Verification items for the finished model (mm, model axes). Coordinates: 2 decimals unless noted, no trailing zeros. Loops run counter-clockwise (first coordinate to the right, second up) from the corner with the lowest first, then second, coordinate; pieces in that order, holes last.
Q1. Sectioned sample at A-A (z = -85). Enter the section's corners in (x, y), then the cut area to 3 significant figures.
Q2. Go/stop test with flat-tipped pins: P1, Ø3, axis at y = 3.5, z = -5, coming from the +X side; P2, Ø3, axis at y = 2, z = -146.5, coming from the +X side; P3, Ø11.5, axis at x = -18, z = -125, coming from the -Y side; P4, Ø5, axis at x = -16.5, z = -84.5, coming from the +Y side. Record where each tip stops, or that it passes through.
Q3. Sectioned sample at D-D (z = -131.5). Enter the section's corners in (x, y).
Q4. Sectioned sample at B-B (y = 2.75). Count the separate pieces of the cut face and the enclosed holes in it, then the cut area to 3 significant figures.
Q5. Sectioned sample at C-C (z = -25). Enter the section's corners in (x, y).
Q6. Material ranges on probe 1 along Z at (x, y) = (-25, 1.1); probe 2 along X at (y, z) = (1.5, -54); probe 3 along X at (y, z) = (1.6, -109), recorded low to high.
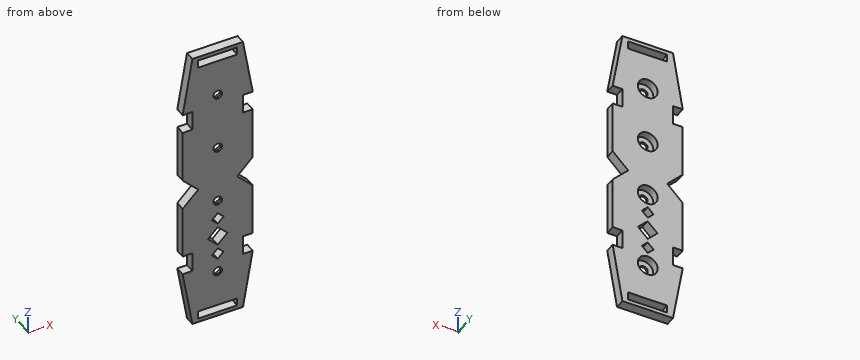
Autodesk Inventor part; units mm, degrees
ref_plane "YZ Plane" through (0, 0, 0) normal (1, 0, 0) x (0, 1, 0)
ref_plane "XZ Plane" through (0, 0, 0) normal (0, 1, 0) x (-1, 0, 0)
ref_plane "XY Plane" through (0, 0, 0) normal (0, 0, 1) x (1, 0, 0)
sketch "Sketch1" plane through (0, 0, 0) normal (0, 1, 0) x (-1, 0, 0)
  line L0 (5, 0) -> (31, 0)
  line L1 (36, -30) -> (36, -120)
  line L2 (31, -150) -> (5, -150)
  line L3 (0, -120) -> (0, -30)
  circle A0 centre (18, -25) radius 5.1
  circle A1 centre (18, -55) radius 5.1
  circle A2 centre (18, -85) radius 5.1
  circle A3 centre (18, -125) radius 5.1
  line L4 (36, -30) -> (31, -30)
  line L5 (31, -30) -> (31, -40)
  line L6 (31, -40) -> (36, -40)
  line L7 (36, -120) -> (31, -120)
  line L8 (31, -120) -> (31, -110)
  line L9 (31, -110) -> (36, -110)
  line L10 (0, -30) -> (5, -30)
  line L11 (5, -30) -> (5, -40)
  line L12 (5, -40) -> (0, -40)
  line L13 (0, -120) -> (5, -120)
  line L14 (5, -120) -> (5, -110)
  line L15 (0, -110) -> (5, -110)
  circle A4 centre (18, -25) radius 2.25
  circle A5 centre (18, -55) radius 2.25
  circle A6 centre (18, -85) radius 2.25
  circle A7 centre (18, -125) radius 2.25
  line L16 (5, 0) -> (0, -30)
  line L17 (31, -150) -> (36, -120)
  line L18 (5, -150) -> (0, -120)
  line L19 (31, 0) -> (36, -30)
  line L20 (18, -100) -> (13, -105)
  line L21 (13, -105) -> (18, -110)
  line L22 (23, -105) -> (18, -110)
  line L23 (23, -105) -> (18, -100)
  line L24 (21, -114.95) -> (18, -117.95)
  line L25 (15, -114.95) -> (18, -117.95)
  line L26 (15, -114.95) -> (18, -111.95)
  line L27 (18, -111.95) -> (21, -114.95)
  line L28 (21, -95.05) -> (18, -98.05)
  line L29 (18, -98.05) -> (15, -95.05)
  line L30 (15, -95.05) -> (18, -92.05)
  line L31 (18, -92.05) -> (21, -95.05)
  line L32 (31, -150) -> (28, -150)
  line L33 (5, -150) -> (8, -150)
  line L34 (8, -148) -> (28, -148)
  line L35 (8, -148) -> (8, -144)
  line L36 (8, -144) -> (28, -144)
  line L37 (28, -144) -> (28, -148)
  line L38 (31, 0) -> (28, 0)
  line L39 (5, 0) -> (8, 0)
  line L40 (8, -2) -> (28, -2)
  line L41 (28, -2) -> (28, -6)
  line L42 (28, -6) -> (8, -6)
  line L43 (8, -6) -> (8, -2)
  line L44 (36, -75) -> (36, -83)
  line L45 (36, -75) -> (36, -67)
  line L46 (36, -67) -> (28, -75)
  line L47 (36, -83) -> (28, -75)
  line L48 (0, -75) -> (0, -83)
  line L49 (0, -75) -> (0, -67)
  line L50 (0, -67) -> (8, -75)
  line L51 (0, -83) -> (8, -75)
  point P0 (0, 0)
  point P1 (18, 0)
  point P2 (18, -150)
  dimension "d2" = 10.2
  dimension "d3" = 25
  dimension "d4" = 10.2
  dimension "d5" = 30
  dimension "d6" = 10.2
  dimension "d7" = 30
  dimension "d8" = 10.2
  dimension "d9" = 40
  dimension "d10" = 25
  dimension "d12" = 5
  dimension "d13" = 10
  dimension "d15" = 10
  dimension "d17" = 5
  dimension "d19" = 5
  dimension "d22" = 4.5
  dimension "d23" = 4.5
  dimension "d24" = 4.5
  dimension "d25" = 4.5
  dimension "d38" = 3
  dimension "d39" = 2
  dimension "d41" = 2
  dimension "d42" = 4
  dimension "d44" = 2
  dimension "d45" = 3
  dimension "d46" = 4
  dimension "d50" = 8
  dimension "d51" = 8
extrude "Extrusion1" add sketch "Sketch1" along normal blind 5 contours L0 L19 L4 L5 L6 L1 L46 L47 L9 L8 L7 L17 L2 L18 L13 L14 L15 L3 L51 L50 L12 L11 L10 L16
extrude "Extrusion2" add sketch "Sketch1" along normal blind 1 contours A0 | A1 | A2 | A3
sketch "Sketch2" plane through (0, 5, 0) normal (0, 1, 0) x (1, 0, 0)
  line L0 (-28, 75) -> (-36, 67)
  line L1 (-36, 110) -> (-36, 83)
  line L2 (-36, 67) -> (-36, 83)
  line L3 (-36, 83) -> (-28, 75)
  line L4 (-36, 83) -> (-28, 75)
  line L5 (-28, 75) -> (-36, 67)
  line L6 (0, 67) -> (-8, 75)
  line L7 (-8, 75) -> (0, 67)
  line L8 (0, 67) -> (0, 83)
  line L9 (0, 83) -> (-8, 75)
  line L10 (-36, 67) -> (0, 67)
  line L11 (-36, 83) -> (0, 83)
  point P0 (0, 0)
properties part number "Side"
Geometry check:
1. outline: (-36, 0) - (-20.25, 0) - (-20.25, 1) - (-23.1, 1) - (-23.1, 5) - (-36, 5) - close; (-15.75, 0) - (0, 0) - (0, 5) - (-12.9, 5) - (-12.9, 1) - (-15.75, 1) - close
1. area: 135 mm2
2. P1: stops at x = -3.92
2. P2: stops at x = -4.17
2. P3: stops at y = 0
2. P4: stops at y = 1
3. outline: (-34.08, 0) - (-1.92, 0) - (-1.92, 5) - (-34.08, 5) - close
4. separate pieces: 1
4. enclosed holes: 9
4. area: 4,200 mm2
5. outline: (-35.17, 0) - (-20.25, 0) - (-20.25, 1) - (-23.1, 1) - (-23.1, 5) - (-35.17, 5) - close; (-15.75, 0) - (-0.83, 0) - (-0.83, 5) - (-12.9, 5) - (-12.9, 1) - (-15.75, 1) - close
6. probe 1: z = -150 to -148, -144 to -6, -2 to 0
6. probe 2: x = -36 to -23, -13 to 0
6. probe 3: x = -36 to -19, -17 to 0
